```python
from build123d import *

# Parameters (mm, degrees)
SKETCH2_W               = 11
SKETCH2_H               = 20
BOSS_EXTRUDE1_DEPTH     = 20
SKETCH3_R               = 15
SKETCH3_R_2             = 9.642090149
CUT_EXTRUDE1_DEPTH      = 42.372377867
CUT_EXTRUDE2_DEPTH      = 42.267785166
CUT_EXTRUDE2_DEPTH_BACK = 42.267785166
SKETCH4_W               = 20
SKETCH4_H               = 4
CUT_EXTRUDE3_DEPTH      = 42.901456055
CUT_EXTRUDE3_DEPTH_BACK = 42.901456055
SKETCH7_R               = 3
CUT_EXTRUDE4_DEPTH      = 44.211230012
SKETCH10_W              = 6
SKETCH10_H              = 6
BOSS_EXTRUDE3_DEPTH     = 18
SKETCH11_R              = 2
CUT_EXTRUDE6_DEPTH      = 39.271928202
SKETCH8_W               = 6
SKETCH8_H               = 6
BOSS_EXTRUDE4_DEPTH     = 18
SKETCH12_R              = 2
CUT_EXTRUDE7_DEPTH      = 46.965327997
SCALE1_SCALE            = 0.75


with BuildPart() as part:
    # Sketch1 → Revolve1 (revolve)
    with BuildSketch(Plane.XY):
        with BuildLine():
            Line((-17.503938211, 9.642090149), (-17.503938211, 0))
            Line((-17.503938211, 0), (20.115058741, 0))
            add(Edge.make_bspline(
                [(-17.503938211, 9.642090149), (-12.037965172, 13.468024809), (1.720669261, 9.986942396), (18.674857326, 10.7604322), (20.115058741, 0)],
                knots=[0, 0, 0, 0, 0.417251545, 1, 1, 1, 1], degree=3))
        make_face()
    revolve(axis=Axis((-34.275157211, 0, 0), (1, 0, 0)))

    # Sketch2 → Boss-Extrude1 (add)
    with BuildSketch(Plane.ZY.offset(17.503938211)):
        Rectangle(SKETCH2_W, SKETCH2_H)
    extrude(amount=BOSS_EXTRUDE1_DEPTH)

    # Sketch3 → Cut-Extrude1 (cut, through all)
    with BuildSketch(Plane.ZY.offset(17.503938211)):
        Circle(SKETCH3_R)
        Circle(SKETCH3_R_2, mode=Mode.SUBTRACT)
    extrude(amount=CUT_EXTRUDE1_DEPTH, mode=Mode.SUBTRACT)

    # Sketch4 → Cut-Extrude2 (cut, two sides: drawn at the far end of the back side and taken through both)
    with BuildSketch(Plane(origin=(0, 0, 0), x_dir=(1, 0, 0), z_dir=(0, 1, 0)).offset(-CUT_EXTRUDE2_DEPTH_BACK)):
        with Locations((-27.503938211, 0)):
            Rectangle(SKETCH4_W, SKETCH4_H)
    extrude(amount=CUT_EXTRUDE2_DEPTH + CUT_EXTRUDE2_DEPTH_BACK, mode=Mode.SUBTRACT)

    # Sketch6 → Cut-Extrude3 (cut, two sides: drawn at the far end of the back side and taken through both)
    with BuildSketch(Plane.XY.offset(-2).offset(-CUT_EXTRUDE3_DEPTH_BACK)):
        with BuildLine():
            Line((-37.503938211, -9.43238583), (-28.071552381, -9.43238583))
            ThreePointArc((-28.071552381, -9.43238583), (-34.741256364, -6.669703983), (-37.503938211, 0))
            Line((-37.503938211, 0), (-37.503938211, -9.43238583))
        make_face()
        with BuildLine():
            Line((-37.503938211, 9.43238583), (-37.503938211, 0))
            ThreePointArc((-37.503938211, 0), (-34.741256364, 6.669703983), (-28.071552381, 9.43238583))
            Line((-28.071552381, 9.43238583), (-37.503938211, 9.43238583))
        make_face()
    extrude(amount=CUT_EXTRUDE3_DEPTH + CUT_EXTRUDE3_DEPTH_BACK, mode=Mode.SUBTRACT)

    # Sketch7 → Cut-Extrude4 (cut, through all)
    with BuildSketch(Plane.XY.offset(5.5)):
        with Locations((-28.071552381, 0)):
            Circle(SKETCH7_R)
    extrude(amount=-CUT_EXTRUDE4_DEPTH, mode=Mode.SUBTRACT)

    # Sketch10 → Boss-Extrude3 (add)
    with BuildSketch(Plane(origin=(0, 0, 0), x_dir=(1, 0, 0), z_dir=(0, 1, 0))):
        with Locations((-9, 0)):
            Rectangle(SKETCH10_W, SKETCH10_H)
    extrude(amount=-BOSS_EXTRUDE3_DEPTH)

    # Sketch11 → Cut-Extrude6 (cut, through all)
    with BuildSketch(Plane(origin=(-6, 0, 0), x_dir=(0, 0, -1), z_dir=(1, 0, 0))):
        with Locations((0, -15.01416918)):
            Circle(SKETCH11_R)
    extrude(amount=-CUT_EXTRUDE6_DEPTH, mode=Mode.SUBTRACT)

    # Sketch8 → Boss-Extrude4 (add)
    with BuildSketch(Plane(origin=(0, 0, 0), x_dir=(1, 0, 0), z_dir=(0, 1, 0))):
        Rectangle(SKETCH8_W, SKETCH8_H)
    extrude(amount=BOSS_EXTRUDE4_DEPTH)

    # Sketch12 → Cut-Extrude7 (cut, through all)
    with BuildSketch(Plane(origin=(3, 0, 0), x_dir=(0, 0, -1), z_dir=(1, 0, 0))):
        with Locations((0, 14.293955788)):
            Circle(SKETCH12_R)
    extrude(amount=-CUT_EXTRUDE7_DEPTH, mode=Mode.SUBTRACT)


with BuildPart() as part_1:
    # Scale1: scaled about (-4.862736276, 0.025056195, 1.7e-08)
    add(part.part.scale(SCALE1_SCALE).moved(Location((-1.215684069, 0.006264049, 4e-09))))


solid = part_1.part
```
Read the model definition and answer for the solid it produces. Units are mm, in the model's axes. A direction names the side the tool comes from. Round coordinates to 2 decimals unless told otherwise and drop trailing zeros. Write each loop counter-clockwise with the first axis right and the second up, starting at its lowest first coordinate (ties: lowest second). Pieces come first, ordered by that corner, then holes. Notation, with made-up numbers: (-25.5, 76.25) - (-5.5, 76.25) arc R15 ccw to (-5.5, 101.25) - close; hole circle Ø10 at (60, 44). An arc over 180 degrees is marked (long way). Use CSV: the item, a comma, the result in double quotes.
Q1. Find section B-B, the plane z = -0.75. Count the separate pieces of the cut face and the enclosed holes in it, then the cut area to 3 significant figures.
Values:
separate pieces,"3"
enclosed holes,"0"
area,"452 mm²"
Q2. Find section A-A, the plane x = -25. Write down the section's boundary in (y, z) (3 decimals).
Values:
outline,"(-6.52, -3.116) arc R7.232 ccw to (-5.933, -4.125) - (5.946, -4.125) arc R7.232 ccw to (6.532, -3.116) - (6.532, -1.5) - (-6.52, -1.5) - close; (-6.52, 1.5) - (6.532, 1.5) - (6.532, 3.116) arc R7.232 ccw to (5.946, 4.125) - (-5.933, 4.125) arc R7.232 ccw to (-6.52, 3.116) - close"
Q3. Determine the mould class of faces 1 (the flat face through (-8, -11, 2.25)), 2 (the cylindrical face through (-7.934, -12.719, 0.325)), 3 (the flat face through (-5.716, -11, 2)), 4 (the flat face through (-1, 11, -2.25)) for opening direction Z: +Z half, -Z half, draft (parallel to the pull), parting line (faces both ways), or undercut.
Values:
face 1,"+Z half"
face 2,"undercut"
face 3,"draft"
face 4,"-Z half"
Q4. A tool of negligible diameter and unlimited length cuts with its end or side. For faces 5 (the flat face through (-14.344, 0, 0)), 6 (the cylindrical face through (-18.84, -6.64, 2.85)), 7 (the cylindrical face through (-20.145, -6.624, -2.888)), from which of +Z, -Z, +X, -X, +Y, -Y can it reach the whole face along a straight path? Write none if from no direction.
Values:
face 5,"-X, +Y, -Y"
face 6,"+Z, -X, -Y"
face 7,"-Z, -X, -Y"
Q5. Each of these flat-tipped pins is pushed along its axis until it touches: pin 1 Ø5 at (y, z) = (-12, 0.5) entering from +X; pin 2 Ø3.5 at (x, y) = (-2, 11) entering from +Z; pin 3 Ø1 at (x, z) = (-20, -3) entering from -Y. Where does it stop, or does it pass through?
Values:
pin 1,"stops at x = -5.72"
pin 2,"stops at z = 2.25"
pin 3,"stops at y = -6.78"
Q6. Straight lines are drawn through the part: line 1 along Z through (x, y) = (-25, -0.75) (3 decimals); line 2 along Y through (x, z) = (-1.3, 0); line 3 along Y through (x, z) = (-0.55, 0). For each, find the intervals that lie inside material, in ascending order.
Values:
line 1,"z = -4.125 to -1.5, 1.5 to 4.125"
line 2,"y = -8.48 to 9.23, 12.23 to 13.51"
line 3,"y = -8.4 to 9.23, 12.23 to 13.51"
